For this review, take the finished solid that the model builds, in its own axes (mm). A direction names the side the tool comes from. Coordinates: 2 decimals unless noted, no trailing zeros. Write each loop counter-clockwise with the first axis right and the second up, starting at its lowest first coordinate (ties: lowest second). Pieces come first, ordered by that corner, then holes. Notation, with made-up numbers: M 88.25,70 L 122.25,70 A22 ccw 122.25,96 Z; hole C 0,-15.5 d2. An arc over 180 degrees is marked long. One line per question, with ' | ' between items.
from build123d import *

# Parameters (mm, degrees)
ESTRUSIONE_ESTRUSIONE1_DEPTH             = 2
RACCORDO1_R                              = 1
RACCORDO2_R                              = 0.5
ESTRUSIONE_ESTRUSIONE2_DEPTH             = 2.5
ESTRUSIONE_ESTRUSIONE2_DEPTH_BACK        = 1.5
SCHIZZO2_R                               = 3
ESTRUSIONE_ESTRUSIONE3_REACH             = 20.547
ESTRUSIONE_ESTRUSIONE3_DIRECTION_2_REACH = 20.547
ESTRUSIONE_ESTRUSIONE4_DEPTH             = 3
RACCORDO3_R                              = 0.5
SCHIZZO5_R                               = 1.5
TAGLIO_ESTRUSIONE1_DEPTH                 = 21.58301689
ESTRUSIONE_ESTRUSIONE5_DEPTH             = 0.1


with BuildPart() as part:
    # Schizzo1 → Estrusione-Estrusione1 (new body)
    with BuildSketch(Plane.XY):
        Polygon((-16.707106781, 0.292893219), (-10.707106781, 0.292893219), (-10, 1), (0, 1), (0, 3), (15, 3), (15, 0), (15, -1.654985921), (9.361844275, -3.707106781), (-11.638155725, -3.707106781), (-11.638155725, -1.707106781), (-16.707106781, -1.707106781), align=None)
    extrude(amount=ESTRUSIONE_ESTRUSIONE1_DEPTH)

    # Raccordo1
    raccordo1_edges = [part.edges().sort_by_distance(p)[0] for p in [
        (-11.638155725, -3.707106781, 1),
    ]]
    fillet(raccordo1_edges, radius=RACCORDO1_R)

    # Raccordo2
    raccordo2_edges = [part.edges().sort_by_distance(p)[0] for p in [
        (-11.638155725, -1.707106781, 1),
    ]]
    fillet(raccordo2_edges, radius=RACCORDO2_R)

    # Schizzo2 → Estrusione-Estrusione2 (add, two sides: drawn at the far end of the back side and taken through both)
    with BuildSketch(Plane.XY.offset(-ESTRUSIONE_ESTRUSIONE2_DEPTH_BACK)):
        with Locations((15, 0)):
            Circle(SCHIZZO2_R)
    extrude(amount=ESTRUSIONE_ESTRUSIONE2_DEPTH + ESTRUSIONE_ESTRUSIONE2_DEPTH_BACK)

    # Estrusione-Estrusione3: up to this face of the body (flat: up to its plane)
    estrusione_estrusione3_end = Plane(part.part.faces().sort_by_distance((0.378494116, -0.704899382, 2))[0])
    # Schizzo3 → Estrusione-Estrusione3 (add, up to the picked face)
    with BuildSketch(Plane.XY, mode=Mode.PRIVATE) as estrusione_estrusione3_sk1:
        with BuildLine():
            Line((18.828427125, 1), (17.828427125, 1))
            ThreePointArc((17.828427125, 1), (18, 0), (17.828427125, -1))
            Line((17.828427125, -1), (18.828427125, -1))
            ThreePointArc((18.828427125, -1), (19.828427125, 0), (18.828427125, 1))
        make_face()
    estrusione_estrusione3_tool1 = split(extrude(estrusione_estrusione3_sk1.sketch, amount=ESTRUSIONE_ESTRUSIONE3_REACH, mode=Mode.PRIVATE), bisect_by=estrusione_estrusione3_end, keep=Keep.BOTH, mode=Mode.PRIVATE)
    add(estrusione_estrusione3_tool1.solids().sort_by(Axis((18.792788, 0, 0), (0, 0, 1)))[0])

    # Estrusione-Estrusione3 direction 2: up to this face of the body (flat: up to its plane)
    estrusione_estrusione3_direction_2_end = Plane(part.part.faces().sort_by_distance((15, 0, -1.5))[0])
    # Schizzo3 → Estrusione-Estrusione3 direction 2 (add, up to the picked face)
    with BuildSketch(Plane.XY, mode=Mode.PRIVATE) as estrusione_estrusione3_direction_2_sk1:
        with BuildLine():
            Line((18.828427125, 1), (17.828427125, 1))
            ThreePointArc((17.828427125, 1), (18, 0), (17.828427125, -1))
            Line((17.828427125, -1), (18.828427125, -1))
            ThreePointArc((18.828427125, -1), (19.828427125, 0), (18.828427125, 1))
        make_face()
    estrusione_estrusione3_direction_2_tool1 = split(extrude(estrusione_estrusione3_direction_2_sk1.sketch, amount=-ESTRUSIONE_ESTRUSIONE3_DIRECTION_2_REACH, mode=Mode.PRIVATE), bisect_by=estrusione_estrusione3_direction_2_end, keep=Keep.BOTH, mode=Mode.PRIVATE)
    add(estrusione_estrusione3_direction_2_tool1.solids().sort_by(Axis((18.792788, 0, 0), (0, 0, -1)))[0])

    # Schizzo4 → Estrusione-Estrusione4 (add)
    with BuildSketch(Plane.ZY.offset(16.707106781)):
        Polygon((2, -1.707106781), (3.5, -1.707106781), (3.5, -3.807106781), (4, -3.807106781), (4, -0.307106781), (2, -0.307106781), align=None)
    extrude(amount=-ESTRUSIONE_ESTRUSIONE4_DEPTH)

    # Raccordo3
    raccordo3_edges = [part.edges().sort_by_distance(p)[0] for p in [
        (-15.207106781, -0.307106781, 4),
        (-13.707106781, -2.057106781, 4),
        (-15.207106781, -3.807106781, 4),
        (-16.707106781, -2.057106781, 4),
    ]]
    fillet(raccordo3_edges, radius=RACCORDO3_R - 0.0001)  # a hair under: the kernel refuses the full size

    # Schizzo5 → Taglio-Estrusione1 (cut, through all)
    with BuildSketch(Plane.XY.offset(2.5)):
        with Locations((15, 0)):
            Circle(SCHIZZO5_R)
    extrude(amount=-TAGLIO_ESTRUSIONE1_DEPTH, mode=Mode.SUBTRACT)

    # Schizzo6 → Estrusione-Estrusione5 (add)
    with BuildSketch(Plane.XY.offset(2)):
        with BuildLine():
            Line((10.5, 1.629867893), (10.5, 0.92944722))
            add(Edge.make_bspline(
                [(10.5, 0.92944722), (10.499844414, 0.882706092), (10.499545672, 0.792957947), (10.497879909, 0.664384677), (10.493105553, 0.54755758), (10.48899697, 0.442537741), (10.481505028, 0.349327086), (10.474344381, 0.267639795), (10.46497072, 0.197852097), (10.456265297, 0.155606246), (10.452323718, 0.13647847)],
                knots=[0, 0, 0, 0, 1.410062039, 2.707475311, 3.878576406, 4.937260626, 5.877586885, 6.699081471, 7.410979367, 8, 8, 8, 8], degree=3))
            add(Edge.make_bspline(
                [(10.452323718, 0.13647847), (10.44599767, 0.110871395), (10.433480527, 0.060203513), (10.407010513, -0.012740009), (10.376429305, -0.082278475), (10.340231746, -0.148150926), (10.299049203, -0.210363472), (10.252641058, -0.268822966), (10.200770974, -0.323195178), (10.144763494, -0.373898474), (10.084129937, -0.419859381), (10.019753567, -0.459632532), (9.952037023, -0.493690082), (9.88074449, -0.520879248), (9.80647863, -0.542752098), (9.72859096, -0.55817975), (9.647429673, -0.567430547), (9.592071808, -0.568372457), (9.564002404, -0.568850055)],
                knots=[0, 0, 0, 0, 1.02737288, 2.032829108, 3.019628684, 3.985738875, 4.958353778, 5.924249254, 6.890702889, 7.883913451, 8.865824512, 9.85161466, 10.829249435, 11.81541824, 12.821369441, 13.843154991, 14.906364023, 16, 16, 16, 16], degree=3))
            add(Edge.make_bspline(
                [(9.564002404, -0.568850055), (9.517367246, -0.567381095), (9.426369973, -0.564514774), (9.294309841, -0.537789138), (9.171117785, -0.494014565), (9.056965246, -0.433684102), (8.954017226, -0.356891178), (8.863900454, -0.264603546), (8.787792734, -0.157292512), (8.735576131, -0.056923958), (8.70197773, 0.031778426), (8.678219098, 0.105018096), (8.660172121, 0.18497086), (8.643769941, 0.270489675), (8.631253759, 0.362235095), (8.622364892, 0.460022369), (8.616649282, 0.564096068), (8.615814207, 0.635435829), (8.615384615, 0.672135521)],
                knots=[0, 0, 0, 0, 1.260402266, 2.459371274, 3.627181936, 4.786749125, 5.93865593, 7.087644312, 8.261344208, 9.485713728, 10.136162886, 10.825977872, 11.566646758, 12.35154167, 13.181268117, 14.0701832, 15.007234106, 16, 16, 16, 16], degree=3))
            Line((8.615384615, 0.672135521), (7, -0.61372185))
            Line((7, -0.61372185), (7, -0.225300376))
            Line((7, -0.225300376), (8.615384615, 1.060556996))
            Line((8.615384615, 1.060556996), (8.615384615, 1.315765329))
            Line((8.615384615, 1.315765329), (7, 1.315765329))
            Line((7, 1.315765329), (7, 1.629867893))
            Line((7, 1.629867893), (10.5, 1.629867893))
        make_face()
        with BuildLine():
            Line((10.141025641, 1.315765329), (8.974358974, 1.315765329))
            Line((8.974358974, 1.315765329), (8.969451122, 0.674940009))
            add(Edge.make_bspline(
                [(8.969451122, 0.674940009), (8.969437885, 0.64501997), (8.969412229, 0.587026413), (8.973406004, 0.503125746), (8.977949327, 0.425005641), (8.984898657, 0.352964869), (8.993854777, 0.286971357), (9.005057604, 0.227057739), (9.01811018, 0.173127354), (9.038309643, 0.110226003), (9.070330282, 0.040008487), (9.116838436, -0.036397556), (9.175714061, -0.101242729), (9.241967426, -0.157151837), (9.316309813, -0.200216089), (9.395441443, -0.23155931), (9.478679147, -0.251228927), (9.53585099, -0.253567367), (9.564703526, -0.254747491)],
                knots=[0, 0, 0, 0, 1.14660753, 2.222451964, 3.218720504, 4.145691244, 4.995719623, 5.770487122, 6.480909919, 7.121111896, 8.299844659, 9.430703709, 10.534634535, 11.641396424, 12.741395289, 13.810956493, 14.895269934, 16, 16, 16, 16], degree=3))
            add(Edge.make_bspline(
                [(9.564703526, -0.254747491), (9.592857905, -0.253563739), (9.648649611, -0.251217974), (9.730103047, -0.231521199), (9.807529909, -0.199713788), (9.879454388, -0.155112436), (9.94528638, -0.101218543), (10.000835297, -0.037211531), (10.047354277, 0.033685128), (10.076864421, 0.09999535), (10.094992971, 0.159223507), (10.107734135, 0.210655613), (10.118056983, 0.268990383), (10.126082803, 0.334088015), (10.133305124, 0.405830736), (10.137987885, 0.484414991), (10.140818147, 0.569750034), (10.140954867, 0.628897216), (10.141025641, 0.659515329)],
                knots=[0, 0, 0, 0, 1.100801541, 2.181386982, 3.260112282, 4.364594493, 5.481957178, 6.577424609, 7.668452592, 8.790448866, 9.403819393, 10.091598921, 10.863153553, 11.720938239, 12.658472417, 13.685008818, 14.801622349, 16, 16, 16, 16], degree=3))
            Line((10.141025641, 0.659515329), (10.141025641, 1.315765329))
        make_face(mode=Mode.SUBTRACT)
    extrude(amount=ESTRUSIONE_ESTRUSIONE5_DEPTH)


solid = part.part
1. Take a section at A-A on z = 0.35. State the section outline as (x, y) points, plus the area to 3 significant figures.
Computed values:
outline: M -16.71,-1.71 L -12.14,-1.71 A0.5 cw -11.64,-2.21 L -11.64,-2.71 A1 ccw -10.64,-3.71 L 9.36,-3.71 L 13.12,-2.34 A3 ccw 17.83,-1 L 18.83,-1 A1 ccw 18.83,1 L 17.83,1 A3 ccw 15,3 L 0,3 L 0,1 L -10,1 L -10.71,0.29 L -16.71,0.29 Z; hole C 15,0 d3 | area: 171 mm2
2. Take a section at B-B on z = -1.05. State the section outline as (x, y) points, plus the area to 3 significant figures.
Computed values:
outline: M 17.83,-1 L 18.83,-1 A1 ccw 18.83,1 L 17.83,1 A3 ccw long Z; hole C 15,0 d3 | area: 24.5 mm2
3. Machinability: for faces 5 (the flat face through (0, 2, 1)), 6 (the flat face through (18, 1, 0)), 7 (the flat face through (-15, -3, 3.5)), 8 (the flat face through (16.3, -1.3, 2.5)), 9 (the flat face through (11.3, -3, 1)), which of the approach directions +Z, -Z, +X, -X, +Y, -Y give a long, thin tool a straight path to every point of the face, cutting with its end or side? Answer none if there is none.
Computed values:
face 5: +Z, -Z, -X, +Y | face 6: +Z, -Z, +X, +Y | face 7: -Z, +X, -X, -Y | face 8: +Z, +X, +Y, -Y | face 9: +Z, -Z, -Y
4. For line 1 along Y through (x, z) = (15, -0.1); line 2 along Z through (x, y) = (11, -1); line 3 along Y through (x, z) = (-8.5, 1.6), list the stretches that pass through material, from the lowest coordinate up.
Computed values:
line 1: y = -3 to -1.5, 1.5 to 3 | line 2: z = 0 to 2 | line 3: y = -3.71 to 1
5. Take a section at C-C on x = -8. State the section outline as (y, z) points.
Computed values:
outline: M -3.71,0 L 1,0 L 1,2 L -3.71,2 Z
6. Clearance check with flat-ended pins moving along their axes: P1, Ø1, axis at x = -14, z = 2, coming from the -Y side; P2, Ø3.5, axis at x = 15, y = 0, coming from the +Z side; P3, Ø0.5, axis at x = -15.5, z = 2.5, coming from the +Y side. State where each tip first meets the part, or that it passes through.
Computed values:
P1: stops at y = -1.71 | P2: stops at z = 2.5 | P3: stops at y = -0.31
7. Draft analysis for pull direction X (two halves, no side actions). For faces 1 (the flat face through (-1, -1, 2)), 2 (the cylindrical face through (-11.34, -3.42, 1.01)), 3 (the flat face through (-14, 0.293, 1)), 4 (the cylindrical face through (13.5, 0.07, 0.53)), state which applies: pulls with the +X half, pulls with the -X half, needs draft (parallel to the pull), parting line crosses it, or undercut.
Computed values:
face 1: undercut | face 2: pulls with the -X half | face 3: needs draft | face 4: undercut
